Geometry: final body of the model. Coordinates: model frame, mm. Face numbers are marked on the shaded views. Give positions to 0.01 mm unless a question says otherwise; leave off trailing zeros. Loops run counter-clockwise (first coordinate to the right, second up) from the corner with the lowest first, then second, coordinate; pieces in that order, holes last.
from build123d import *

# Parameters (mm, degrees)
MASTER_FOOTPRINT_W    = 1350
MASTER_FOOTPRINT_H    = 700
BATH_BASE_PLATE_DEPTH = 750
BATH_SHELL_2MM_T      = -2


with BuildPart() as part:
    # MASTER_FOOTPRINT → BATH_BASE_PLATE (new body)
    with BuildSketch(Plane(origin=(0, 0, 0), x_dir=(1, 0, 0), z_dir=(0, 1, 0))):
        with Locations((675, 350)):
            Rectangle(MASTER_FOOTPRINT_W, MASTER_FOOTPRINT_H)
    extrude(amount=BATH_BASE_PLATE_DEPTH)

    # BATH_SHELL_2MM
    bath_shell_2mm_openings = [part.faces().sort_by_distance(p)[0] for p in [
        (675, 750, -350),
    ]]
    offset(amount=BATH_SHELL_2MM_T, openings=bath_shell_2mm_openings, kind=Kind.INTERSECTION)


solid = part.part
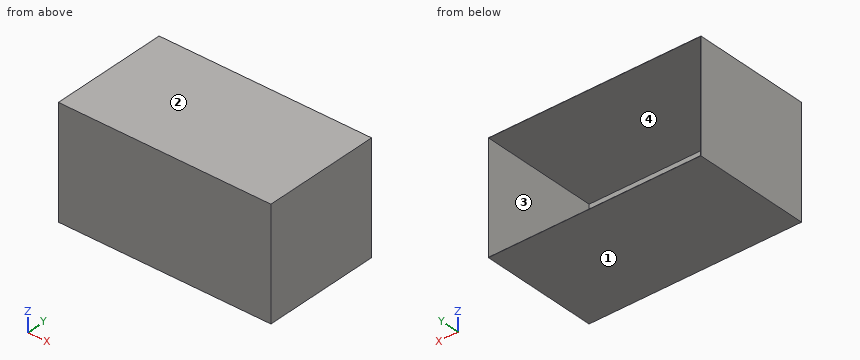
Item 1: Draft query along Z for the marked faces 1, 2, 3 and 4. Return one class per face: +Z half, -Z half, draft (parallel to the pull), parting line (faces both ways), or undercut.
Values follow:
face 1: -Z half
face 2: +Z half
face 3: undercut
face 4: undercut
Item 2: Ray query, probe 1 along Z at (x, y) = (220.5, 60); probe 2 along X at (y, z) = (262, -173.5); probe 3 along Y at (x, z) = (473, -563.5). Return the intervals inside material, ascending.
Values follow:
probe 1: z = -700 to -698, -2 to 0
probe 2: x = 0 to 2, 1348 to 1350
probe 3: y = 0 to 2
Item 3: Pin query (flat end, axial travel): pin 1 (6 mm diameter, centred on x = 480, z = -589.5, fed in from +Y). Return the tip coordinate at first contact, or that it passes through.
Values follow:
pin 1: stops at y = 2
Item 4: Section query B-B on x = 346. Return loops of the section in (y, z), plus the area to 3 significant figures.
Values follow:
outline: (0, -700) - (750, -700) - (750, -698) - (2, -698) - (2, -2) - (750, -2) - (750, 0) - (0, 0) - close
area: 4,390 mm2
Item 5: Section query A-A on y = 693. Return loops of the section in (x, z).
Values follow:
outline: (0, -700) - (1350, -700) - (1350, 0) - (0, 0) - close; hole (2, -698) - (1348, -698) - (1348, -2) - (2, -2) - close
Item 6: Section query C-C on z = -99.5. Return loops of the section in (x, y), plus the area to 3 significant figures.
Values follow:
outline: (0, 0) - (1350, 0) - (1350, 750) - (1348, 750) - (1348, 2) - (2, 2) - (2, 750) - (0, 750) - close
area: 5,690 mm2
